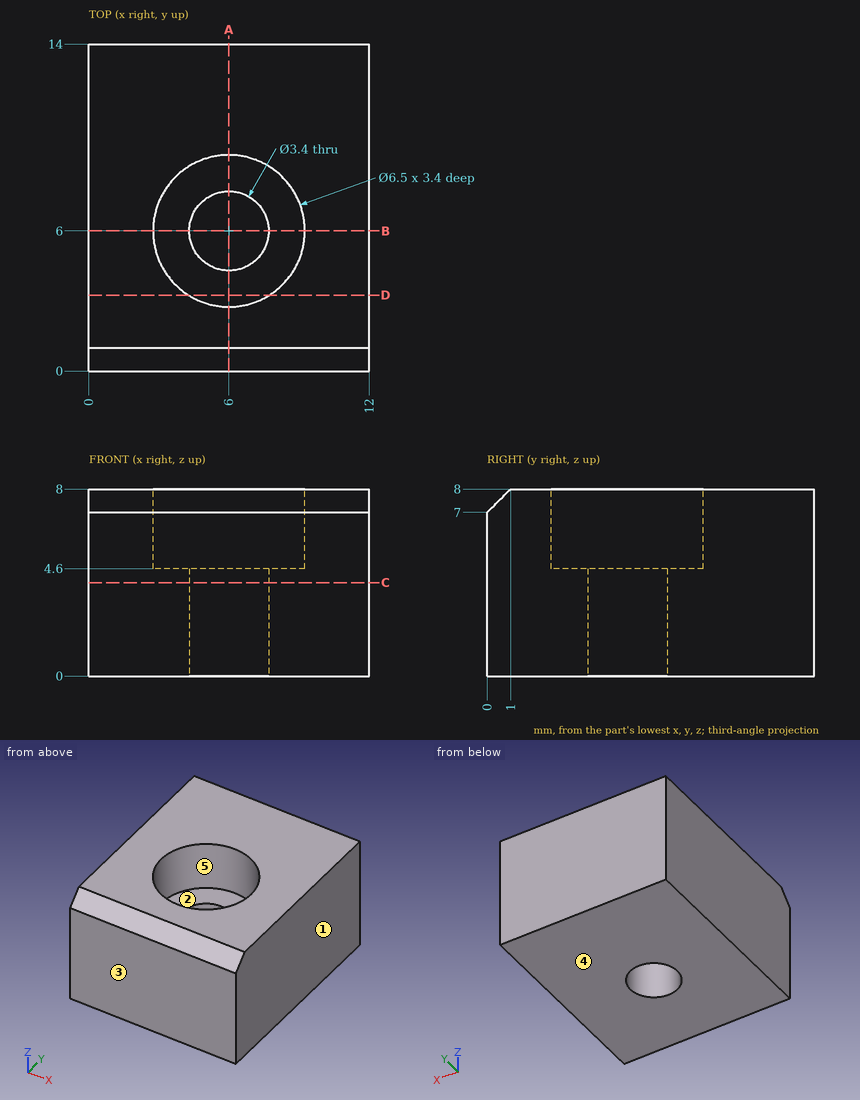
Geometry: see drawing. Coordinates: mm, zero at the bounding-box minimum. A direction names the side the tool comes from. Give positions to 0.01 mm unless a question says otherwise; leave off trailing zeros. Loops run counter-clockwise (first coordinate to the right, second up) from the corner with the lowest first, then second, coordinate; pieces in that order, holes last. Notation, with made-up numbers: (68, -15.5) -> (118, -15.5) arc R16 cw to (118, -0.5) -> close; hole circle Ø6 at (-29.5, -4.5). An arc over 180 degrees is marked (long way). Use one line per item in the form item = value.
Item 1: Access query for the marked faces 1 and 2. Directions: +Z, -Z, +X, -X, +Y, -Y. A direction counts if a zero-diameter tool reaches every point of the face in a straight line with its end or side. Return the directions, or none.
A:
face_1 = +Z, -Z, +X, +Y, -Y
face_2 = +Z
Item 2: Pin query (flat end, axial travel): P1, Ø3, axis at x = 5.5, y = 7.5, coming from the +Z side. Return the tip coordinate at first contact, or that it passes through.
A:
P1 = 4.6
Item 3: Draft query along Y for the marked faces 3, 4 and 5. Return one class per face: pulls with the +Y half, pulls with the -Y half, needs draft (parallel to the pull), parting line crosses it, or undercut.
A:
face_3 = pulls with the -Y half
face_4 = needs draft
face_5 = undercut
Item 4: Section query A-A on x = 6. Output: boundary loops of the cut face in (y, z).
A:
outline = (0, 0) -> (4.3, 0) -> (4.3, 4.6) -> (2.75, 4.6) -> (2.75, 8) -> (1, 8) -> (0, 7) -> close; (7.7, 0) -> (14, 0) -> (14, 8) -> (9.25, 8) -> (9.25, 4.6) -> (7.7, 4.6) -> close
Item 5: Line query: probe 1 along Y at (x, z) = (6, 3.5); probe 2 along Y at (x, z) = (6, 6); probe 3 along X at (y, z) = (4.75, 7.75). Output: solid intervals per line, ascending.
A:
probe_1 = 0 to 4.3, 7.7 to 14
probe_2 = 0 to 2.75, 9.25 to 14
probe_3 = 0 to 3, 9 to 12
Item 6: Section query D-D on y = 3.25. Output: boundary loops of the cut face in (x, z).
A:
outline = (0, 0) -> (12, 0) -> (12, 8) -> (7.73, 8) -> (7.73, 4.6) -> (4.27, 4.6) -> (4.27, 8) -> (0, 8) -> close
Item 7: Section query B-B on y = 6. Output: boundary loops of the cut face in (x, z), and give its area (3 significant figures).
A:
outline = (0, 0) -> (4.3, 0) -> (4.3, 4.6) -> (2.75, 4.6) -> (2.75, 8) -> (0, 8) -> close; (7.7, 0) -> (12, 0) -> (12, 8) -> (9.25, 8) -> (9.25, 4.6) -> (7.7, 4.6) -> close
area = 58.3 mm^2
Item 8: Section query C-C on z = 4. Output: boundary loops of the cut face in (x, y), and give its area (3 significant figures).
A:
outline = (0, 0) -> (12, 0) -> (12, 14) -> (0, 14) -> close; hole circle Ø3.4 at (6, 6)
area = 159 mm^2
